```python
from build123d import *

# Parameters (mm, degrees)
HEX_NUT_DEPTH         = 13
SKETCH2_R             = 10.4775
THREAD_BORE_DEPTH     = 11
PUSH_FIT_PORT_START   = 13
SKETCH3_R             = 6
PUSH_FIT_PORT_DEPTH   = 12
PUSH_FIT_SOCKET_START = 25
SKETCH4_R             = 3.2
PUSH_FIT_SOCKET_DEPTH = 10


with BuildPart() as part:
    # Sketch1 → Hex_Nut (new body)
    with BuildSketch(Plane.XY):
        Polygon((12, 6.92820323), (0, 13.856406461), (-12, 6.92820323), (-12, -6.92820323), (0, -13.856406461), (12, -6.92820323), align=None)
    extrude(amount=HEX_NUT_DEPTH)

    # Sketch2 → Thread_Bore (cut)
    with BuildSketch(Plane.XY):
        Circle(SKETCH2_R)
    extrude(amount=THREAD_BORE_DEPTH, mode=Mode.SUBTRACT)

    # Sketch3 → Push_Fit_Port (add)
    with BuildSketch(Plane.XY.offset(PUSH_FIT_PORT_START)):
        Circle(SKETCH3_R)
    extrude(amount=PUSH_FIT_PORT_DEPTH)

    # Sketch4 → Push_Fit_Socket (cut)
    with BuildSketch(Plane.XY.offset(PUSH_FIT_SOCKET_START)):
        Circle(SKETCH4_R)
    extrude(amount=-PUSH_FIT_SOCKET_DEPTH, mode=Mode.SUBTRACT)


solid = part.part
```
CAD build for the part. Positions are in the model's coordinates, mm. A direction names the side the tool comes from. Coordinates: 2 decimals unless noted, no trailing zeros. Write each loop counter-clockwise with the first axis right and the second up, starting at its lowest first coordinate (ties: lowest second). Pieces come first, ordered by that corner, then holes. Notation, with made-up numbers: (-24, -35) -> (0, -35) arc R5 ccw to (0, -27) -> close; hole circle Ø8 at (71.5, 39). An arc over 180 degrees is marked (long way). Return JSON: item names as keys, results as strings. Group by question number.
Q1. Which spindle directions (+Z, -Z, +X, -X, +Y, -Y) get a long thin tool onto all of the face, cutting with end or side? Do faces 1 (the face through (-6, -3, 13)), 2 (the face through (-1.36, 10.39, 5.42)), 3 (the face through (3, -3, 25)). Say none if no direction does.
Q2. Cut at B-B, the plane z = 4.5. Give the cut face in (x, y) (1 decimal).
Q3. Drill centre lines: line 1 (Y direction, x = 0, z = 8); line 2 (Y direction, x = 0, z = 22); line 3 (Z direction, x = -4.75, y = -6). Where is each one in solid material? Low to high.
Q4. Cut at D-D, the plane x = -4. Give the cut face in (y, z).
Q5. Pull direction Y, two halves, no side cores. Call faces 4 (the face through (-6.084, -10.344, 6.409)), 5 (the face through (0, 0, 15)), 6 (the face through (12, 0, 6)), 7 (the face through (-6, 0, 19)): released by +Y, released by -Y, zero draft, split by the parting line, or undercut.
Q6. Flat gauge pins, fed straight in: pin 1 (8 mm diameter, centred on x = -3, z = 19.5, fed in from -Y); pin 2 (3 mm diameter, centred on x = 2.5, z = 10.5, fed in from -Y); pin 3 (6 mm diameter, centred on x = -8, z = 5.5, fed in from -Y). Where does each tip first touch, or does it go through?
Q7. Cut at C-C, the plane z = 12.25. Give the cut face in (x, y).
Q8. Cut at A-A, the plane y = 0. Give the cut face in (x, z).
Returned:
{
 "1": {"face 1": "+Z", "face 2": "-Z", "face 3": "+Z, +X, -X, +Y, -Y"},
 "2": {"outline": "(-12, -6.9) -> (0, -13.9) -> (12, -6.9) -> (12, 6.9) -> (0, 13.9) -> (-12, 6.9) -> close; hole circle Ø21 at (0, 0)"},
 "3": {"line 1": "y = -13.86 to -10.48, 10.48 to 13.86", "line 2": "y = -6 to -3.2, 3.2 to 6", "line 3": "z = 11 to 13"},
 "4": {"outline": "(-11.55, 0) -> (-9.68, 0) -> (-9.68, 11) -> (9.68, 11) -> (9.68, 0) -> (11.55, 0) -> (11.55, 13) -> (4.47, 13) -> (4.47, 25) -> (-4.47, 25) -> (-4.47, 13) -> (-11.55, 13) -> close"},
 "5": {"face 4": "released by -Y", "face 5": "undercut", "face 6": "zero draft", "face 7": "split by the parting line"},
 "6": {"pin 1": "stops at y = -6", "pin 2": "stops at y = -13.28", "pin 3": "stops at y = -10.97"},
 "7": {"outline": "(-12, -6.93) -> (0, -13.86) -> (12, -6.93) -> (12, 6.93) -> (0, 13.86) -> (-12, 6.93) -> close"},
 "8": {"outline": "(-12, 0) -> (-10.48, 0) -> (-10.48, 11) -> (10.48, 11) -> (10.48, 0) -> (12, 0) -> (12, 13) -> (6, 13) -> (6, 25) -> (3.2, 25) -> (3.2, 15) -> (-3.2, 15) -> (-3.2, 25) -> (-6, 25) -> (-6, 13) -> (-12, 13) -> close"}
}
